from build123d import *

# Parameters (mm, degrees)
PLATE_START      = 92.57
PLATE_SKETCH_W   = 90
PLATE_SKETCH_H   = 50
PLATE_SKETCH_R   = 2.2
PLATE_SKETCH_R_2 = 1.7
PLATE_DEPTH      = 3.18
PADS_START       = 95.75
PADS_SKETCH_R    = 4
PADS_SKETCH_R_2  = 2.2
PADS_DEPTH       = 3.3


with BuildPart() as part:
    # Plate Sketch → Plate (new body)
    with BuildSketch(Plane(origin=(0, 0, 0), x_dir=(1, 0, 0), z_dir=(0, 1, 0)).offset(PLATE_START)):
        Rectangle(PLATE_SKETCH_W, PLATE_SKETCH_H)
        with Locations(Location((-37, 0, 0), (0, 0, 270))):
            Circle(PLATE_SKETCH_R, mode=Mode.SUBTRACT)
        with Locations(Location((37, 0, 0), (0, 0, 270))):
            Circle(PLATE_SKETCH_R, mode=Mode.SUBTRACT)
        with Locations(Location((-31.25, 9.25, 0), (0, 0, 270))):
            Circle(PLATE_SKETCH_R_2, mode=Mode.SUBTRACT)
        with Locations(Location((31.25, -9.25, 0), (0, 0, 270))):
            Circle(PLATE_SKETCH_R_2, mode=Mode.SUBTRACT)
    extrude(amount=PLATE_DEPTH)

    # Pads Sketch → Pads (add)
    # profile 1 of 2: a face of its own
    with BuildSketch(Plane(origin=(0, 0, 0), x_dir=(1, 0, 0), z_dir=(0, 1, 0)).offset(PADS_START)):
        with Locations(Location((-37, 0, 0), (0, 0, 90))):
            Circle(PADS_SKETCH_R)
        with Locations(Location((-37, 0, 0), (0, 0, 270))):
            Circle(PADS_SKETCH_R_2, mode=Mode.SUBTRACT)
    # profile 2 of 2: a face of its own
    with BuildSketch(Plane(origin=(0, 0, 0), x_dir=(1, 0, 0), z_dir=(0, 1, 0)).offset(PADS_START)):
        with Locations(Location((37, 0, 0), (0, 0, 90))):
            Circle(PADS_SKETCH_R)
        with Locations(Location((37, 0, 0), (0, 0, 270))):
            Circle(PADS_SKETCH_R_2, mode=Mode.SUBTRACT)
    extrude(amount=PADS_DEPTH)


solid = part.part
The model under review builds one solid part; all positions refer to its coordinate system, in mm. A direction names the side the tool comes from. Give positions to 0.01 mm unless a question says otherwise; leave off trailing zeros. Order: outer loops, then holes, each group sorted by start corner. A loop starts at its lowest first (then second) coordinate and runs counter-clockwise, first axis right, second up. Notation, with made-up numbers: (67, -18) -> (95, -18) arc R30 cw to (95, 15) -> close; hole circle Ø4 at (83.25, 39.5). An arc over 180 degrees is marked (long way). Write item = value, one per line. Start each with the question number.
(1) Draft analysis for pull direction Z (two halves, no side actions). For faces 1 (the flat face through (-45, 94, 0)), 2 (the cylindrical face through (-39.148, 95.765, -0.477)), 3 (the flat face through (-1, 94, -25)), 4 (the cylindrical face through (-32.91, 94.14, -9.62)), state which applies: +Z half, -Z half, draft (parallel to the pull), parting line (faces both ways), or undercut.
(2) Take a section at C-C (y = 96.75). Write out the cut boundary in (x, z), plus the area to 3 significant figures.
(3) Tool access review of faces 5 (the flat face through (-35, 99.05, -2)), 6 (the cylindrical face through (-40.966, 97.377, 0.521)): name each direction out of +Z, -Z, +X, -X, +Y, -Y from which nothing blocks a thin tool from reaching the whole face with its end or side.
(4) For L1, parallel to X at y = 94.5, z = 0; L2, parallel to X at y = 94.3, z = 9.25; L3, parallel to X at y = 93.8, z = -9.25, list the stretches that pass through material, from the lowest coordinate up. Write a range as from..to.
(5) For pin 1 Ø5 at (x, z) = (-31, -13.5) entering from +Y, flat-tipped, find the tip position at first contact; note if it passes through.
(6) Take a section at D-D (z = -9.25). Write out the cut boundary in (x, y).
(7) Take a section at A-A (z = 0). Write out the cut boundary in (x, y), plus the area to 3 significant figures.
(8) Take a section at B-B (x = -31.25). Write out the cut boundary in (y, z).
Returned:
q1.face_1 = draft
q1.face_2 = undercut
q1.face_3 = -Z half
q1.face_4 = undercut
q2.outline = circle Ø8 at (-37, 0); circle Ø8 at (37, 0); hole circle Ø4.4 at (-37, 0); hole circle Ø4.4 at (37, 0)
q2.area = 70.1 mm²
q3.face_5 = +Z, -Z, +X, -X, +Y
q3.face_6 = +Y
q4.L1 = -45..-39.2, -34.8..34.8, 39.2..45
q4.L2 = -45..29.55, 32.95..45
q4.L3 = -45..-32.95, -29.55..45
q5.pin_1 = 95.75
q6.outline = (-45, 92.57) -> (-32.95, 92.57) -> (-32.95, 95.75) -> (-45, 95.75) -> close; (-29.55, 92.57) -> (45, 92.57) -> (45, 95.75) -> (-29.55, 95.75) -> close
q7.outline = (-45, 92.57) -> (-39.2, 92.57) -> (-39.2, 99.05) -> (-41, 99.05) -> (-41, 95.75) -> (-45, 95.75) -> close; (-34.8, 92.57) -> (34.8, 92.57) -> (34.8, 99.05) -> (33, 99.05) -> (33, 95.75) -> (-33, 95.75) -> (-33, 99.05) -> (-34.8, 99.05) -> close; (39.2, 92.57) -> (45, 92.57) -> (45, 95.75) -> (41, 95.75) -> (41, 99.05) -> (39.2, 99.05) -> close
q7.area = 282 mm²
q8.outline = (92.57, -25) -> (95.75, -25) -> (95.75, -10.95) -> (92.57, -10.95) -> close; (92.57, -7.55) -> (95.75, -7.55) -> (95.75, 25) -> (92.57, 25) -> close
